```python
from build123d import *

# Parameters (mm, degrees)
SKETCH1_W           = 173.99
SKETCH1_H           = 38.1
BOSS_EXTRUDE1_DEPTH = 3.175
SKETCH2_W           = 15.875
SKETCH2_H           = 3.175
SKETCH2_W_2         = 12.7
SKETCH2_W_3         = 3.175
SKETCH2_H_2         = 12.7
CUT_EXTRUDE1_DEPTH  = 3.175


with BuildPart() as part:
    # Sketch1 → Boss-Extrude1 (new body)
    with BuildSketch(Plane(origin=(0, 0, 0), x_dir=(1, 0, 0), z_dir=(0, 1, 0))):
        Rectangle(SKETCH1_W, SKETCH1_H)
    extrude(amount=BOSS_EXTRUDE1_DEPTH)

    # Sketch2 → Cut-Extrude1 (cut)
    with BuildSketch(Plane(origin=(0, 3.175, 0), x_dir=(1, 0, 0), z_dir=(0, 1, 0))):
        with Locations((-79.0575, 17.4625)):
            Rectangle(SKETCH2_W, SKETCH2_H)
        with Locations((-52.07, 17.4625)):
            Rectangle(SKETCH2_W_2, SKETCH2_H)
        with Locations((-26.67, 17.4625)):
            Rectangle(SKETCH2_W_2, SKETCH2_H)
        with Locations((-1.27, 17.4625)):
            Rectangle(SKETCH2_W_2, SKETCH2_H)
        with Locations((24.13, 17.4625)):
            Rectangle(SKETCH2_W_2, SKETCH2_H)
        with Locations((49.53, 17.4625)):
            Rectangle(SKETCH2_W_2, SKETCH2_H)
        Polygon((68.58, 19.05), (68.58, 15.875), (81.28, 15.875), (86.995, 15.875), (86.995, 19.05), (81.28, 19.05), align=None)
        with Locations((-85.4075, 0)):
            Rectangle(SKETCH2_W_3, SKETCH2_H_2)
        with Locations((85.4075, 0)):
            Rectangle(SKETCH2_W_3, SKETCH2_H_2)
    extrude(amount=-CUT_EXTRUDE1_DEPTH, mode=Mode.SUBTRACT)


solid = part.part
```
Source: CAD feature listing. Evaluate the final solid. Frame: model axes, mm. A direction names the side the tool comes from. Coordinates: 2 decimals unless noted, no trailing zeros. Loops run counter-clockwise (first coordinate to the right, second up) from the corner with the lowest first, then second, coordinate; pieces in that order, holes last. Notation, with made-up numbers: M -13,37.5 L 5,37.5 A23 cw 5,50.5 Z; hole C 54,-3 d3. An arc over 180 degrees is marked long. Use CSV: the item, a comma, the result in double quotes.
(1) Line query: line 1 (X direction, y = 0.55, z = -17); line 2 (X direction, y = 0.6, z = 0); line 3 (Z direction, x = -76, y = 0.65) (3 decimals). Output: solid intervals per line, ascending. Write a range as [from, to].
Answers follow:
line 1,"[-71.12, -58.42], [-45.72, -33.02], [-20.32, -7.62], [5.08, 17.78], [30.48, 43.18], [55.88, 68.58]"
line 2,"[-83.82, 83.82]"
line 3,"[-15.875, 19.05]"
(2) Cut plane A-A on z = 0.5. Return loops of the section in (x, y) (3 decimals).
Answers follow:
outline,"M -83.82,0 L 83.82,0 L 83.82,3.175 L -83.82,3.175 Z"
(3) Draft query along X for faces 5 (the face through (-86.995, 2, -11)), 6 (the face through (-20.32, 2, -17)), 7 (the face through (37, 2, -19.05)), 8 (the face through (-33.02, 2, -17)). Return one class per face: pulls with the +X half, pulls with the -X half, needs draft (parallel to the pull), parting line crosses it, or undercut.
Answers follow:
face 5,"pulls with the -X half"
face 6,"undercut"
face 7,"needs draft"
face 8,"undercut"
(4) Reachability of faces 1 (the face through (-71.12, 2, -17)), 2 (the face through (-83.82, 2, 0)), 3 (the face through (78, 2, -15.875)), 4 (the face through (-58.42, 2, -17)) from +Z, -Z, +X, -X, +Y, -Y: full face, straight path, thin tool, end or side. Return the list, or none.
Answers follow:
face 1,"-Z, -X, +Y, -Y"
face 2,"-X, +Y, -Y"
face 3,"-Z, +X, +Y, -Y"
face 4,"-Z, +Y, -Y"
(5) Contact query for flat-ended pins moving along their axis: pin 1 (1.6 mm diameter, centred on x = 85.5, y = 2, fed in from -Z) (3 decimals); pin 2 (1 mm diameter, centred on y = 2, z = -18, fed in from -X); pin 3 (1.6 mm diameter, centred on y = 2, z = 1, fed in from -X). Output: stop coordinate, or through.
Answers follow:
pin 1,"z = -15.875"
pin 2,"x = -71.12"
pin 3,"x = -83.82"
(6) Cut plane B-B on x = 50.5. Return loops of the section in (y, z) (3 decimals), and give its area (3 significant figures).
Answers follow:
outline,"M 0,-15.875 L 3.175,-15.875 L 3.175,19.05 L 0,19.05 Z"
area,"111 mm²"
